The drawing under review shows one solid part. Ordinate dimensions are in mm from its lowest x, y, z. Round coordinates to 2 decimals unless told otherwise and drop trailing zeros. Order: outer loops, then holes, each group sorted by start corner. A loop starts at its lowest first (then second) coordinate and runs counter-clockwise, first axis right, second up. Notation, with made-up numbers: M 64.5,10 L 70.5,10 A28 ccw 70.5,34 Z; hole C 58,34.5 d3. An arc over 180 degrees is marked long. Answer as a JSON object with one key per item and string values. Group by question number.
1) Consider section B-B, the plane z = 175.8. Write out the cut boundary in (x, y).
2) Consider section C-C, the plane y = 15.75. Write out the cut boundary in (x, z), then the cut area to 3 significant figures.
3) Consider section A-A, the plane x = 175.8. Write out the cut boundary in (y, z).
4) The part is to be moulded in two halves that separate along Z. For the marked faces 1 and 2, say which applies: +Z half, -Z half, draft (parallel to the pull), parting line (faces both ways), or undercut.
5) To check wall thickness, follow line 1 (Z direction, x = 177.5, y = 18.5); line 2 (X direction, y = 2, z = 241); line 3 (Y direction, x = 179.5, z = 209.5). State the ranges of each line that lie inside material, in increasing order.
6) Insertion check: pin 1 Ø8 at (x, y) = (174, 4.5) entering from +Z; pin 2 Ø1 at (x, y) = (193.5, 10.5) entering from -Z; pin 3 Ø5 at (y, z) = (6, 104.5) entering from +X. Each pin has a flat end and moves straight along its axis. Give the tip position at first contact, or say it passes through.
7) Consider section D-D, the plane x = 295. Write out the cut boundary in (y, z).
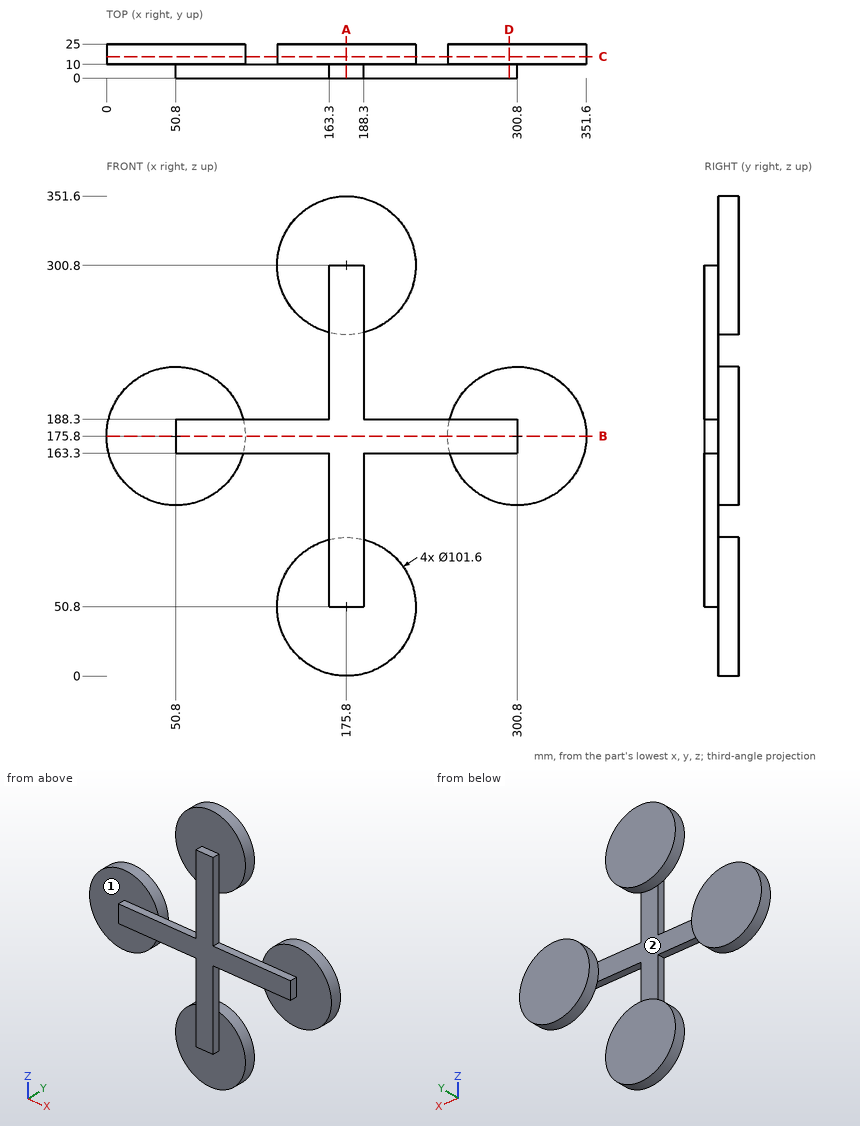
Results list:
{
 "1": {"outline": "M 0,10 L 50.8,10 L 50.8,0 L 300.8,0 L 300.8,10 L 351.6,10 L 351.6,25 L 250,25 L 250,10 L 101.6,10 L 101.6,25 L 0,25 Z"},
 "2": {"outline": "C 50.8,175.8 d101.6; C 175.8,50.8 d101.6; C 175.8,300.8 d101.6; C 300.8,175.8 d101.6", "area": "32,400 mm^2"},
 "3": {"outline": "M 0,50.8 L 10,50.8 L 10,0 L 25,0 L 25,101.6 L 10,101.6 L 10,250 L 25,250 L 25,351.6 L 10,351.6 L 10,300.8 L 0,300.8 Z"},
 "4": {"face 1": "draft", "face 2": "undercut"},
 "5": {"line 1": "0.03 to 101.57, 250.03 to 351.57", "line 2": "163.3 to 188.3", "line 3": "0 to 10"},
 "6": {"pin 1": "z = 300.8", "pin 2": "z = 3", "pin 3": "x = 188.3"},
 "7": {"outline": "M 0,163.3 L 10,163.3 L 10,125.33 L 25,125.33 L 25,226.27 L 10,226.27 L 10,188.3 L 0,188.3 Z"}
}
